The drawing under review shows one solid part. Ordinate dimensions are in mm from its lowest x, y, z. Coordinates: 2 decimals unless noted, no trailing zeros. Order: outer loops, then holes, each group sorted by start corner. A loop starts at its lowest first (then second) coordinate and runs counter-clockwise, first axis right, second up. Notation, with made-up numbers: (28, 74) -> (66, 74) arc R9 cw to (66, 91) -> close; hole circle Ø4 at (38, 86). An arc over 180 degrees is marked (long way). Use one line per item in the form item = value.
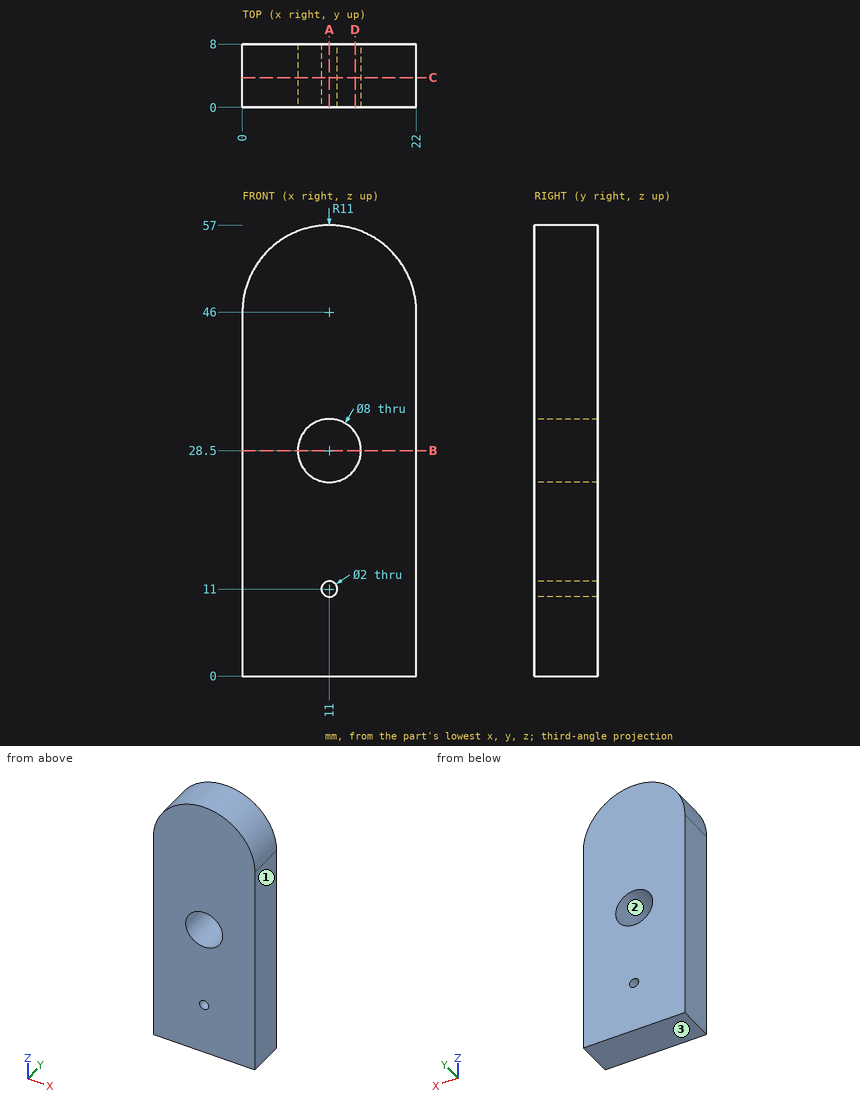
Item 1: We need section C-C (y = 3.75). Write out the cut boundary in (x, z).
Results found:
outline = (0, 0) -> (22, 0) -> (22, 46) arc R11 ccw to (0, 46) -> close; hole circle Ø8 at (11, 28.5); hole circle Ø2 at (11, 11)
Item 2: We need section A-A (x = 11). Write out the cut boundary in (y, z), plus the area to 3 significant figures.
Results found:
outline = (0, 0) -> (8, 0) -> (8, 10) -> (0, 10) -> close; (0, 12) -> (8, 12) -> (8, 24.5) -> (0, 24.5) -> close; (0, 32.5) -> (8, 32.5) -> (8, 57) -> (0, 57) -> close
area = 376 mm²
Item 3: We need section D-D (x = 14.25). Write out the cut boundary in (y, z), plus the area to 3 significant figures.
Results found:
outline = (0, 0) -> (8, 0) -> (8, 26.17) -> (0, 26.17) -> close; (0, 30.83) -> (8, 30.83) -> (8, 56.51) -> (0, 56.51) -> close
area = 415 mm²
Item 4: Draft analysis for pull direction Z (two halves, no side actions). For the marked faces 1, 2 and 3, state which applies: released by +Z, released by -Z, zero draft, split by the parting line, or undercut.
Results found:
face_1 = zero draft
face_2 = undercut
face_3 = released by -Z
Item 5: We need section B-B (z = 28.5). Write out the cut boundary in (x, y).
Results found:
outline = (0, 0) -> (7, 0) -> (7, 8) -> (0, 8) -> close; (15, 0) -> (22, 0) -> (22, 8) -> (15, 8) -> close
Item 6: Clearance check with a flat-ended pin moving along its axis: pin 1 (2 mm diameter, centred on x = 16.5, y = 1.5, fed in from +Z). State where the tip first meets the part, or that it passes through.
Results found:
pin_1 = 56.04
Item 7: To check wall thickness, follow L1, parallel to Z at x = 11, y = 5.5; L2, parallel to Z at x = 9, y = 1; L3, parallel to X at y = 1, z = 26. State the ranges of each line that lie inside material, in increasing order. Write a range as from..to.
Results found:
L1 = 0..10, 12..24.5, 32.5..57
L2 = 0..25.04, 31.96..56.82
L3 = 0..7.88, 14.12..22
